```python
from build123d import *

# Parameters (mm, degrees)
BOSS_EXTRUDE1_DEPTH = 1.2
CUT_EXTRUDE2_DEPTH  = 2.2


with BuildPart() as part:
    # Sketch1 → Boss-Extrude1 (new body)
    with BuildSketch(Plane(origin=(0, 0, 0), x_dir=(1, 0, 0), z_dir=(0, 1, 0))):
        with BuildLine():
            Line((3.748031496, 8.025459318), (5.748031496, 8.025459318))
            Line((5.748031496, 8.025459318), (5.748031496, -10.904540682))
            Line((5.748031496, -10.904540682), (3.748031496, -10.904540682))
            ThreePointArc((3.748031496, -10.904540682), (3.040924715, -11.197433901), (2.748031496, -11.904540682))
            Line((2.748031496, -11.904540682), (2.748031496, -13.904540682))
            Line((2.748031496, -13.904540682), (-8.751968504, -13.904540682))
            Line((-8.751968504, -13.904540682), (-8.751968504, -11.904540682))
            ThreePointArc((-8.751968504, -11.904540682), (-9.751968504, -10.904540682), (-10.751968504, -11.904540682))
            Line((-10.751968504, -11.904540682), (-10.751968504, -13.904540682))
            Line((-10.751968504, -13.904540682), (-18.051968504, -13.904540682))
            Line((-18.051968504, -13.904540682), (-18.051968504, 11.025459318))
            Line((-18.051968504, 11.025459318), (-10.751968504, 11.025459318))
            Line((-10.751968504, 11.025459318), (-10.751968504, 9.025459318))
            ThreePointArc((-10.751968504, 9.025459318), (-9.751968504, 8.025459318), (-8.751968504, 9.025459318))
            Line((-8.751968504, 9.025459318), (-8.751968504, 11.025459318))
            Line((-8.751968504, 11.025459318), (2.748031496, 11.025459318))
            Line((2.748031496, 11.025459318), (2.748031496, 9.025459318))
            ThreePointArc((2.748031496, 9.025459318), (3.040924715, 8.318352536), (3.748031496, 8.025459318))
        make_face()
    extrude(amount=BOSS_EXTRUDE1_DEPTH)

    # Sketch2 → Cut-Extrude2 (cut, through all)
    with BuildSketch(Plane(origin=(0, 1.2, 0), x_dir=(1, 0, 0), z_dir=(0, 1, 0))):
        with BuildLine():
            Line((-4.351968504, 7.175459318), (-4.351968504, 11.025459318))
            Line((-4.351968504, 11.025459318), (-0.751968504, 11.025459318))
            Line((-0.751968504, 11.025459318), (-0.751968504, 7.175459318))
            ThreePointArc((-0.751968504, 7.175459318), (-2.551968504, 5.375459318), (-4.351968504, 7.175459318))
        make_face()
    cut_extrude2 = extrude(amount=-CUT_EXTRUDE2_DEPTH, mode=Mode.SUBTRACT)

    # Mirror2: Cut-Extrude2 across plane
    add(cut_extrude2.mirror(Plane.XY.offset(1.439540682)), mode=Mode.SUBTRACT)


solid = part.part
```
Read the model definition and answer for the solid it produces. Units are mm, in the model's axes. A direction names the side the tool comes from. Coordinates: 2 decimals unless noted, no trailing zeros. Order: outer loops, then holes, each group sorted by start corner. A loop starts at its lowest first (then second) coordinate and runs counter-clockwise, first axis right, second up. Notation, with made-up numbers: (56.5, 70) - (97.5, 70) arc R15 ccw to (97.5, 91) - close; hole circle Ø10 at (78.5, 81.5). An arc over 180 degrees is marked (long way). Answer as a JSON object with one key per item and string values. Group by question number.
Item 1: Section A-A (y = 0.8) is taken. Give the vertices of the cut face in (x, z).
Item 2: Flat-ended cylindrical pins translate along their axes: P1, Ø0.6, axis at y = 0.5, z = 12, coming from the +X side; P2, Ø0.6, axis at y = 0.5, z = 13.5, coming from the +X side; P3, Ø0.6, axis at x = 4.5, y = 0.5, coming from the -Z side; P4, Ø8, axis at x = -2.5, z = 8, coming from the -Y side. Find the tip coordinate at first contact, or state that the pin passes through.
Item 3: A tool of negligible diameter and unlimited length cuts with its end or side. For faces 1 (the face through (5, 1, -8.025)), 2 (the face through (-10.752, 1, -10)), 3 (the face through (1, 1, -11.025)), from which of +Z, -Z, +X, -X, +Y, -Y can it reach the whole face along a straight path? Write none if from no direction.
Item 4: Section C-C (x = 3.25) is taken. Give the vertices of the cut face in (y, z).
Item 5: Section B-B (z = -6.5) is taken. Give the vertices of the cut face in (x, y), plus the area to 3 significant figures.
Item 6: Consider probe 1 along X at (y, z) = (0.8, -9); probe 2 along X at (y, z) = (0.6, -7.75); probe 3 along X at (y, z) = (0.95, 9.25). Determine where each line is inside the solid, lowest interval first. Write a range as from..to.
Item 7: The mould has two halves that part along X. Classify faces 4 (the face through (-14, 1, 13.905)), 5 (the face through (-4.352, 1, -9)), 6 (the face through (2.748, 1, 13)): +X half, -X half, draft (parallel to the pull), parting line (faces both ways), or undercut.
Item 8: Section D-D (x = -9.5) is taken. Give the vertices of the cut face in (y, z).
Results are:
{
 "1": {"outline": "(-18.05, -11.03) - (-10.75, -11.03) - (-10.75, -9.03) arc R1 cw to (-8.75, -9.03) - (-8.75, -11.03) - (-4.35, -11.03) - (-4.35, -7.18) arc R1.8 cw to (-0.75, -7.18) - (-0.75, -11.03) - (2.75, -11.03) - (2.75, -9.03) arc R1 cw to (3.75, -8.03) - (5.75, -8.03) - (5.75, 10.9) - (3.75, 10.9) arc R1 cw to (2.75, 11.9) - (2.75, 13.9) - (-0.75, 13.9) - (-0.75, 10.05) arc R1.8 cw to (-4.35, 10.05) - (-4.35, 13.9) - (-8.75, 13.9) - (-8.75, 11.9) arc R1 cw to (-10.75, 11.9) - (-10.75, 13.9) - (-18.05, 13.9) - close"},
 "2": {"P1": "stops at x = 2.77", "P2": "stops at x = 2.75", "P3": "stops at z = -8.03", "P4": "stops at y = 0"},
 "3": {"face 1": "-Z, +X, +Y, -Y", "face 2": "-Z, +Y, -Y", "face 3": "-Z, +X, -X, +Y, -Y"},
 "4": {"outline": "(0, -8.16) - (1.2, -8.16) - (1.2, 11.04) - (0, 11.04) - close"},
 "5": {"outline": "(-18.05, 0) - (-4.22, 0) - (-4.22, 1.2) - (-18.05, 1.2) - close; (-0.88, 0) - (5.75, 0) - (5.75, 1.2) - (-0.88, 1.2) - close", "area": "24.6 mm^2"},
 "6": {"probe 1": "x = -18.05..-10.75, -8.75..-4.35, -0.75..2.75", "probe 2": "x = -18.05..-4.35, -0.75..5.75", "probe 3": "x = -18.05..-4.16, -0.94..5.75"},
 "7": {"face 4": "draft", "face 5": "undercut", "face 6": "+X half"},
 "8": {"outline": "(0, -8.06) - (1.2, -8.06) - (1.2, 10.94) - (0, 10.94) - close"}
}
